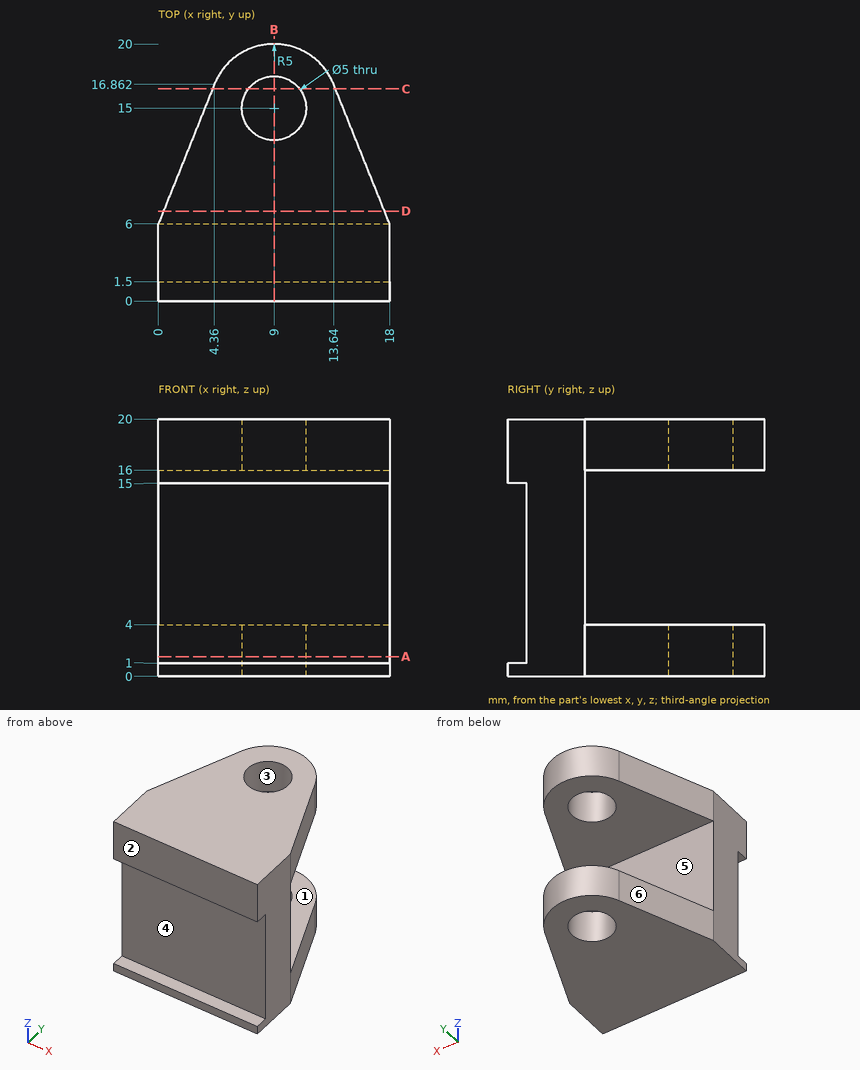
Geometry: see drawing. Coordinates: mm, zero at the bounding-box minimum. A direction names the side the tool comes from. Round coordinates to 2 decimals unless told otherwise and drop trailing zeros. Loops run counter-clockwise (first coordinate to the right, second up) from the corner with the lowest first, then second, coordinate; pieces in that order, holes last. Notation, with made-up numbers: M 19.25,13.25 L 60.25,13.25 A24 cw 60.25,28.25 Z; hole C -23.5,8 d6. An arc over 180 degrees is marked long. Use a Markdown table: item, result. Add a question column.
1. Mould query, pull axis Y, two halves, no side actions, for the marked faces 1, 2 and 3. Classes: pulls with the +Y half, pulls with the -Y half, needs draft (parallel to the pull), parting line crosses it, or undercut.
2. Section query D-D on y = 7. Return the cut outline in (x, z), then the cut area to 3 significant figures.
3. Section query B-B on x = 9. Return the cut outline in (y, z).
4. Line query: line 1 (Z direction, x = 11.75, y = 11); line 2 (Y direction, x = 9, z = 17.05); line 3 (Y direction, x = 9, z = 1.4). Output: solid intervals per line, ascending.
5. Contact query for flat-ended pins moving along their axis: P1, Ø6, axis at x = 6, z = 8, coming from the +Y side; P2, Ø1, axis at x = 9.5, y = 13.5, coming from the -Z side; P3, Ø1, axis at x = 9, z = 6, coming from the -Y side. Output: stop coordinate, or through.
6. Section query C-C on y = 16.5. Return the cut outline in (x, z) (1 decimal).
7. Reachability of the marked faces 4, 5 and 6 from +Z, -Z, +X, -X, +Y, -Y: full face, straight path, thin tool, end or side. Return the list, or none.
8. Section query A-A on z = 1.5. Return the cut outline in (x, y).
Reported:
| question | item | result |
|---|---|---|
| 1 | face 1 | needs draft |
| 1 | face 2 | pulls with the -Y half |
| 1 | face 3 | undercut |
| 2 | outline | M 0.4,0 L 17.6,0 L 17.6,4 L 0.4,4 Z; M 0.4,16 L 17.6,16 L 17.6,20 L 0.4,20 Z |
| 2 | area | 138 mm² |
| 3 | outline | M 0,0 L 12.5,0 L 12.5,4 L 6,4 L 6,16 L 12.5,16 L 12.5,20 L 0,20 L 0,15 L 1.5,15 L 1.5,1 L 0,1 Z; M 17.5,0 L 20,0 L 20,4 L 17.5,4 Z; M 17.5,16 L 20,16 L 20,20 L 17.5,20 Z |
| 4 | line 1 | z = 0 to 4, 16 to 20 |
| 4 | line 2 | y = 0 to 12.5, 17.5 to 20 |
| 4 | line 3 | y = 1.5 to 12.5, 17.5 to 20 |
| 5 | P1 | stops at y = 6 |
| 5 | P2 | passes through |
| 5 | P3 | stops at y = 1.5 |
| 6 | outline | M 4.2,0 L 7,0 L 7,4 L 4.2,4 Z; M 4.2,16 L 7,16 L 7,20 L 4.2,20 Z; M 11,0 L 13.8,0 L 13.8,4 L 11,4 Z; M 11,16 L 13.8,16 L 13.8,20 L 11,20 Z |
| 7 | face 4 | +X, -X, -Y |
| 7 | face 5 | +X, -X, +Y |
| 7 | face 6 | +Z, -Z, -X, +Y |
| 8 | outline | M 0,1.5 L 18,1.5 L 18,6 L 13.64,16.86 A5 ccw 4.36,16.86 L 0,6 Z; hole C 9,15 d5 |
